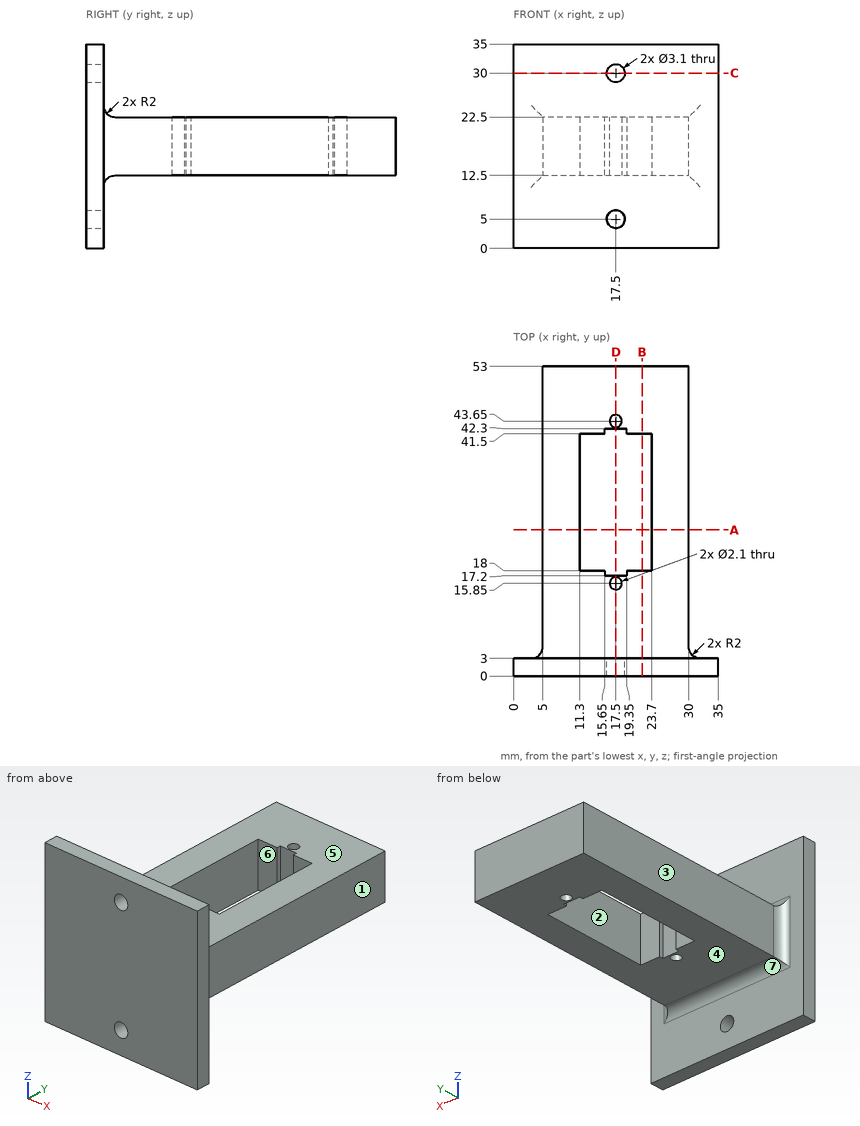
Print and shaded views of the part. All mm, measured from the part's lowest x, y and z. A direction names the side the tool comes from. Give positions to 0.01 mm unless a question says otherwise; leave off trailing zeros. Write each loop counter-clockwise with the first axis right and the second up, starting at its lowest first coordinate (ties: lowest second). Pieces come first, ordered by that corner, then holes. Notation, with made-up numbers: M 8,-2 L 59,-2 A30 ccw 59,35 Z; hole C 68.5,51.5 d11. An arc over 180 degrees is marked long. Use a Markdown table: item, result.
1) Cut at C-C (z = 30). List the corners of the cut face in (x, y), and give its area (3 significant figures).
Responses:
| item | result |
|---|---|
| outline | M 0,0 L 15.95,0 L 15.95,3 L 0,3 Z; M 19.05,0 L 35,0 L 35,3 L 19.05,3 Z |
| area | 95.7 mm2 |
2) Cut at A-A (y = 25). List the corners of the cut face in (x, z).
Responses:
| item | result |
|---|---|
| outline | M 5,12.5 L 11.3,12.5 L 11.3,22.5 L 5,22.5 Z; M 23.7,12.5 L 30,12.5 L 30,22.5 L 23.7,22.5 Z |
3) Drill centre lines: line 1 (Z direction, x = 17.5, y = 0.8); line 2 (Y direction, x = 17.5, z = 18.25); line 3 (Y direction, x = 23, z = 13). Where is each one in solid material? Low to high. Write a range as from..to.
Responses:
| item | result |
|---|---|
| line 1 | z = 0..3.45, 6.55..28.45, 31.55..35 |
| line 2 | y = 0..14.8, 16.9..17.2, 42.3..42.6, 44.7..53 |
| line 3 | y = 0..18, 41.5..53 |
4) Pull direction Y, two halves, no side cores. Call the marked faces 5, 6 and 7: +Y half, -Y half, draft (parallel to the pull), parting line (faces both ways), or undercut.
Responses:
| item | result |
|---|---|
| face 5 | draft |
| face 6 | undercut |
| face 7 | +Y half |
5) Cut at B-B (x = 22). List the corners of the cut face in (y, z).
Responses:
| item | result |
|---|---|
| outline | M 0,0 L 3,0 L 3,10.5 A2 cw 5,12.5 L 18,12.5 L 18,22.5 L 5,22.5 A2 cw 3,24.5 L 3,35 L 0,35 Z; M 41.5,12.5 L 53,12.5 L 53,22.5 L 41.5,22.5 Z |
6) Tool access for the marked faces 1, 2, 3 and 4: list every direction of +Z, -Z, +X, -X, +Y, -Y with a clear straight run to the whole face (end or side of a thin tool).
Responses:
| item | result |
|---|---|
| face 1 | +Z, -Z, +X, +Y |
| face 2 | +Z, -Z |
| face 3 | +Z, -Z, -X, +Y |
| face 4 | -Z, +X, -X, +Y |
7) Pin check, flat tips, straight feed: pin 1 (1.5 mm diameter, centred on y = 11, z = 19, fed in from +X); pin 2 (3 mm diameter, centred on x = 16, z = 31, fed in from +Y); pin 3 (2 mm diameter, centred on x = 6.5, y = 42, fed in from +Z). Stop position of each tip, or through.
Responses:
| item | result |
|---|---|
| pin 1 | stops at x = 30 |
| pin 2 | stops at y = 3 |
| pin 3 | stops at z = 22.5 |
8) Cut at D-D (x = 17.5). Give the number of separate pieces and of enclosed holes in the cut face, and give its area (3 significant figures).
Responses:
| item | result |
|---|---|
| separate pieces | 6 |
| enclosed holes | 0 |
| area | 295 mm2 |
